Input: part model. Units: mm. Frame: model coordinates. A direction names the side the tool comes from. Coordinates: 2 decimals unless noted, no trailing zeros. Write each loop counter-clockwise with the first axis right and the second up, starting at its lowest first coordinate (ties: lowest second). Pieces come first, ordered by that corner, then holes. Notation, with made-up numbers: M 3.5,65.25 L 56.5,65.25 A6 ccw 56.5,72.25 Z; hole C -21,25 d2. An arc over 180 degrees is marked long. Use CSV: the item, a comma, the result in double quotes.
```python
from build123d import *

# Parameters (mm, degrees)
SKETCH1_W                    = 25.4
SKETCH1_H                    = 25.4
SKETCH1_W_2                  = 19.05
SKETCH1_H_2                  = 19.05
BOSS_EXTRUDE1_DEPTH          = 203.2
CUT_EXTRUDE1_DEPTH           = 206.174779152
F_3_8_0_375_DIAMETER_HOLE1_D = 9.525


with BuildPart() as part:
    # Sketch1 → Boss-Extrude1 (new body)
    with BuildSketch(Plane.XY):
        Rectangle(SKETCH1_W, SKETCH1_H)
        Rectangle(SKETCH1_W_2, SKETCH1_H_2, mode=Mode.SUBTRACT)
    extrude(amount=BOSS_EXTRUDE1_DEPTH)

    # Sketch2 → Cut-Extrude1 (cut, through all)
    with BuildSketch(Plane(origin=(12.7, 0, 0), x_dir=(0, 0, -1), z_dir=(1, 0, 0))):
        Polygon((0, 12.7), (0, -12.7), (-25.4, 12.7), align=None)
    extrude(amount=-CUT_EXTRUDE1_DEPTH, mode=Mode.SUBTRACT)

    # 3/8 (0.375) Diameter Hole1 (through all)
    with Locations(Plane(origin=(0, -12.7, 0), x_dir=(-1, 0, 0), z_dir=(0, -1, 0))):
        with Locations((0, -190.5)):
            Hole(F_3_8_0_375_DIAMETER_HOLE1_D / 2)


solid = part.part
```
1. Section A-A (y = -5.25). Return loops of the section in (x, z) (3 decimals).
Resolved:
outline,"M -12.7,7.45 L -9.525,7.45 L -9.525,203.2 L -12.7,203.2 Z; M 9.525,7.45 L 12.7,7.45 L 12.7,203.2 L 9.525,203.2 Z"
2. Material intervals for line 1 (X direction, y = 6.5, z = 58.5) (3 decimals); line 2 (X direction, y = -11.8, z = 190.5), sorted ascending. Write a range as [from, to].
Resolved:
line 1,"x = [-12.7, -9.525], [9.525, 12.7]"
line 2,"x = [-12.7, -4.76], [4.76, 12.7]"
3. Access query for faces 1 (the flat face through (9.525, 0, 102)), 2 (the flat face through (0, -12.7, 100)). Directions: +Z, -Z, +X, -X, +Y, -Y. A direction counts if a zero-diameter tool reaches every point of the face in a straight line with its end or side. Return the directions, or none.
Resolved:
face 1,"+Z, -Z"
face 2,"+Z, -Z, +X, -X, -Y"
4. Section C-C (z = 190.5). Return loops of the section in (x, y) (1 decimal).
Resolved:
outline,"M -12.7,-12.7 L -4.8,-12.7 L -4.8,-9.5 L -9.5,-9.5 L -9.5,9.5 L -4.8,9.5 L -4.8,12.7 L -12.7,12.7 Z; M 4.8,-12.7 L 12.7,-12.7 L 12.7,12.7 L 4.8,12.7 L 4.8,9.5 L 9.5,9.5 L 9.5,-9.5 L 4.8,-9.5 Z"
5. Section B-B (x = 7.25). Return loops of the section in (y, z) (3 decimals), then the cut area to 3 significant figures.
Resolved:
outline,"M -12.7,0 L -9.525,3.175 L -9.525,203.2 L -12.7,203.2 Z; M 9.525,22.225 L 12.7,25.4 L 12.7,203.2 L 9.525,203.2 Z"
area,"1,210 mm^2"
6. Section D-D (z = 150). Return loops of the section in (x, y) (3 decimals), then the cut area to 3 significant figures.
Resolved:
outline,"M -12.7,-12.7 L 12.7,-12.7 L 12.7,12.7 L -12.7,12.7 Z; hole M -9.525,-9.525 L 9.525,-9.525 L 9.525,9.525 L -9.525,9.525 Z"
area,"282 mm^2"
7. Mould query, pull axis Y, two halves, no side actions, for faces 3 (the flat face through (-11.1, -0.2, 12.5)), 4 (the flat face through (0, 9.525, 111)), 5 (the cylindrical face through (-1.03, -11.09, 195.15)). Classes: pulls with the +Y half, pulls with the -Y half, needs draft (parallel to the pull), parting line crosses it, or undercut.
Resolved:
face 3,"pulls with the +Y half"
face 4,"undercut"
face 5,"needs draft"
